The drawing under review shows one solid part. Ordinate dimensions are in mm from its lowest x, y, z. A direction names the side the tool comes from. Give positions to 0.01 mm unless a question says otherwise; leave off trailing zeros. Write each loop counter-clockwise with the first axis right and the second up, starting at its lowest first coordinate (ties: lowest second). Pieces come first, ordered by that corner, then holes.
Q1. We need section C-C (z = 14). Write out the cut boundary in (x, y), then the cut area to 3 significant figures.
Q2. We need section A-A (x = 150). Write out the cut boundary in (y, z).
Q3. Machinability: for the marked faces 1, 2 and 3, which of the approach directions +Z, -Z, +X, -X, +Y, -Y give a long, thin tool a straight path to every point of the face, cutting with its end or side? Answer none if there is none.
Q4. Insertion check: P1, Ø3.5, axis at y = 37.5, z = 8, coming from the -X side; P2, Ø6, axis at y = 28.5, z = 3, coming from the +X side; P3, Ø5, axis at x = 137.5, z = 13, coming from the -Y side. Each pin has a flat end and moves straight along its axis. Give the tip position at first contact, or say it passes through.
Q5. For line 1 (Y direction, x = 160, z = 16.25); line 2 (X direction, y = 55.5, z = 9.75); line 3 (X direction, y = 17, z = 17.75), list the stretches that pass through material, from the lowest coordinate up.
Q6. We need section B-B (y = 42). Write out the cut boundary in (x, z).
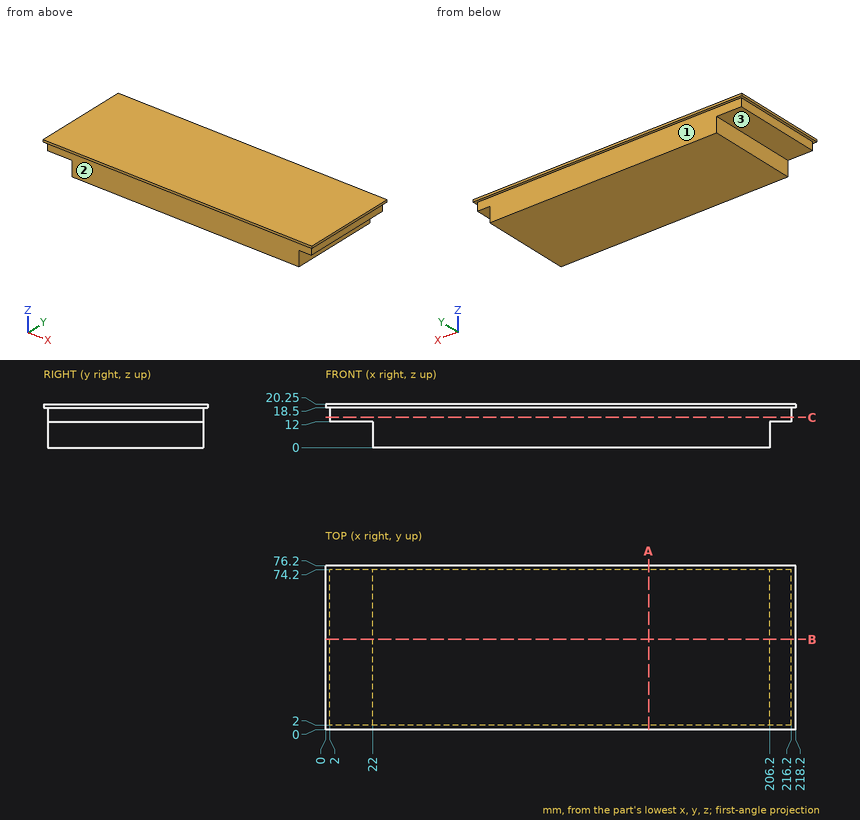
Computed:
1. outline: (2, 2) - (216.2, 2) - (216.2, 74.2) - (2, 74.2) - close
1. area: 15,500 mm2
2. outline: (0, 18.5) - (2, 18.5) - (2, 0) - (74.2, 0) - (74.2, 18.5) - (76.2, 18.5) - (76.2, 20.25) - (0, 20.25) - close
3. face 1: -Z, +X, -X, +Y
3. face 2: -Z, +X, -X, -Y
3. face 3: -Z, -X, +Y, -Y
4. P1: stops at x = 22
4. P2: stops at x = 206.2
4. P3: stops at y = 2
5. line 1: y = 2 to 74.2
5. line 2: x = 22 to 206.2
5. line 3: x = 2 to 216.2
6. outline: (0, 18.5) - (2, 18.5) - (2, 12) - (22, 12) - (22, 0) - (206.2, 0) - (206.2, 12) - (216.2, 12) - (216.2, 18.5) - (218.2, 18.5) - (218.2, 20.25) - (0, 20.25) - close
